Geometry: final body of the model. Coordinates: model frame, mm. A direction names the side the tool comes from. Coordinates: 2 decimals unless noted, no trailing zeros. Write each loop counter-clockwise with the first axis right and the second up, starting at its lowest first coordinate (ties: lowest second). Pieces come first, ordered by that corner, then holes. Notation, with made-up numbers: (9, 55) - (22, 55) arc R22 ccw to (22, 84) - close; hole circle Ø4 at (4.5, 74). An arc over 180 degrees is marked (long way). Answer as a JSON object with one key per item and string values. Group by question number.
Item 1: Section C-C on z = 17.5. Return loops of the section in (x, y), and give its area (3 significant figures).
Item 2: Section D-D on y = -209. Return loops of the section in (x, z), and give its area (3 significant figures).
Item 3: Set-up query: faces 5 (the flat face through (39, -125, 10)), 6 (the flat face through (1, -124, 20)). Return all of +Z, -Z, +X, -X, +Y, -Y with unobstructed straight access to the full face (end or side cutting, diameter ignored); none if empty.
Item 4: Section A-A on x = -15. Return loops of the section in (y, z).
Item 5: Line query: line 1 along Y through (x, z) = (-15, 5.75); line 2 along Y through (x, z) = (33.5, 9.5); line 3 along Z through (x, y) = (-33, -15). Output: solid intervals per line, ascending. Write a range as from..to.
Item 6: Mould query, pull axis X, two halves, no side actions, for faces 1 (the cylindrical face through (35.716, -123.547, 4.93)), 2 (the cylindrical face through (36.19, -214.37, 4.93)), 3 (the cylindrical face through (-30.3, -12, 8.4)), 4 (the flat face through (-47, -2, 10)). Classes: pulls with the +X half, pulls with the -X half, needs draft (parallel to the pull), parting line crosses it, or undercut.
Item 7: Section B-B on y = -15. Return loops of the section in (x, z), and give its area (3 significant figures).
Item 8: First-contact query: pin 1 Ø5.5 at (x, y) = (38, -206) entering from +Z; pin 2 Ø14.5 at (x, y) = (32.5, -130.5) entering from +Z; pin 3 Ø10 at (x, z) = (5, 16.5) entering from +Y; pin 4 Ø9 at (x, y) = (35, -209) entering from +Z. Flat tips, straight axial feed; report the tip coordinate or a pass-through.
```python
from build123d import *

# Parameters (mm, degrees)
SKETCH_3_W                    = 20
SKETCH_3_H                    = 244
EXTRUDE_1_DEPTH               = 50
SKETCH_4_W                    = 60
SKETCH_4_H                    = 20
CUT_EXTRUDE_1_DEPTH           = 34
HOLE_WIZARD_M8_1_D            = 6.8
CHAMFER_1_SIZE                = 60
CHAMFER_2_SIZE                = 5
HOLE_WIZARD_M10_1_D           = 11
HOLE_WIZARD_M10_1_CBORE_D     = 18
HOLE_WIZARD_M10_1_CBORE_DEPTH = 10
HOLE_WIZARD_8_0_8_1_D         = 8
FILLET_1_DEPTH                = 20


with BuildPart() as part:
    # 草圖3 → 伸長1 (new, symmetric)
    with BuildSketch(Plane(origin=(0, 0, 0), x_dir=(0, 0, -1), z_dir=(1, 0, 0))):
        with Locations((-10, -122)):
            Rectangle(SKETCH_3_W, SKETCH_3_H)
    extrude(amount=EXTRUDE_1_DEPTH, both=True)

    # 草圖4 → 除料-伸長1 (cut)
    with BuildSketch(Plane(origin=(0, 0, 0), x_dir=(1, 0, 0), z_dir=(0, 1, 0))):
        with Locations((20, -10)):
            Rectangle(SKETCH_4_W, SKETCH_4_H)
    extrude(amount=-CUT_EXTRUDE_1_DEPTH, mode=Mode.SUBTRACT)

    # M8 螺紋孔1 (through all)
    with Locations(Plane(origin=(-10, -84.062632567, -21.444178573), x_dir=(0, 0, 1), z_dir=(1, 0, 0))):
        with Locations((31.444178573, -69.062632567)):
            Hole(HOLE_WIZARD_M8_1_D / 2)

    # 導角1
    chamfer_1_edges = [part.edges().sort_by_distance(p)[0] for p in [
        (50, -34, 10),
    ]]
    chamfer(chamfer_1_edges, length=CHAMFER_1_SIZE - 0.0001)  # a hair under: the kernel refuses the full size

    # 導角2
    chamfer_2_edges = [part.edges().sort_by_distance(p)[0] for p in [
        (-50, 0, 10),
        (-50, -244, 10),
        (50, -244, 10),
    ]]
    chamfer(chamfer_2_edges, length=CHAMFER_2_SIZE)

    # M10 六角承窩頭蓋螺釘的柱孔1 (through all)
    with Locations(Plane.XY.offset(20)):
        with Locations((-15, -129), (35, -129), (-15, -209), (35, -209)):
            CounterBoreHole(HOLE_WIZARD_M10_1_D / 2, HOLE_WIZARD_M10_1_CBORE_D / 2, HOLE_WIZARD_M10_1_CBORE_DEPTH)

    # Ø8.0 (8) 直徑孔1 (through all)
    with Locations(Plane.XY.offset(20)):
        with Locations((10, -129), (10, -209)):
            Hole(HOLE_WIZARD_8_0_8_1_D / 2)

    # 圓角1: read off the stored shape, not the designer's step
    # 圓角1 outline → 圓角1 (add)
    with BuildSketch(Plane.XY):
        with BuildLine():
            ThreePointArc((-8.535533906, -35.464466094), (-9.619397663, -33.84234935), (-10, -31.928932188))
            Line((-10, -31.928932188), (-10, -34))
            Line((-10, -34), (-8.535533906, -35.464466094))
        make_face()
    extrude(amount=FILLET_1_DEPTH)


solid = part.part
```
Checks:
{
 "1": {"outline": "(-50, -239) - (-45, -244) - (45, -244) - (50, -239) - (50, -94) - (-8.55, -35.45) arc R5 cw to (-10, -31.93) - (-10, 0) - (-45, 0) - (-50, -5) - close; hole circle Ø18 at (-15, -209); hole circle Ø18 at (-15, -129); hole circle Ø8 at (10, -209); hole circle Ø8 at (10, -129); hole circle Ø18 at (35, -209); hole circle Ø18 at (35, -129)", "area": "19,400 mm^2"},
 "2": {"outline": "(-50, 0) - (-20.5, 0) - (-20.5, 10) - (-24, 10) - (-24, 20) - (-50, 20) - close; (-9.5, 0) - (6, 0) - (6, 20) - (-6, 20) - (-6, 10) - (-9.5, 10) - close; (14, 0) - (29.5, 0) - (29.5, 10) - (26, 10) - (26, 20) - (14, 20) - close; (40.5, 0) - (50, 0) - (50, 20) - (44, 20) - (44, 10) - (40.5, 10) - close", "area": "1,260 mm^2"},
 "3": {"face 5": "+Z", "face 6": "+Z, +X, -X, +Y, -Y"},
 "4": {"outline": "(-244, 0) - (-214.5, 0) - (-214.5, 10) - (-218, 10) - (-218, 20) - (-244, 20) - close; (-203.5, 0) - (-134.5, 0) - (-134.5, 10) - (-138, 10) - (-138, 20) - (-200, 20) - (-200, 10) - (-203.5, 10) - close; (-123.5, 0) - (0, 0) - (0, 20) - (-120, 20) - (-120, 10) - (-123.5, 10) - close; hole circle Ø6.8 at (-15, 10)"},
 "5": {"line 1": "-244..-214.5, -203.5..-134.5, -123.5..0", "line 2": "-244..-214.29, -203.71..-134.29, -123.71..-77.5", "line 3": "0..6.6, 13.4..20"},
 "6": {"face 1": "undercut", "face 2": "undercut", "face 3": "needs draft", "face 4": "pulls with the -X half"},
 "7": {"outline": "(-50, 0) - (-10, 0) - (-10, 6.6) - (-50, 6.6) - close; (-50, 13.4) - (-10, 13.4) - (-10, 20) - (-50, 20) - close", "area": "528 mm^2"},
 "8": {"pin 1": "z = 10", "pin 2": "z = 20", "pin 3": "y = -44", "pin 4": "through"}
}
